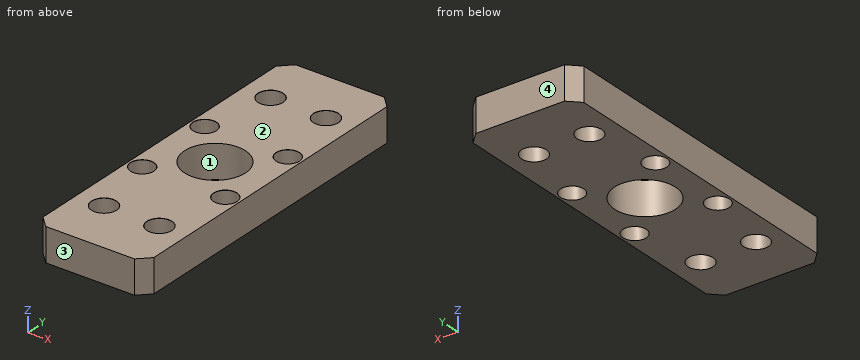
```python
from build123d import *

# Parameters (mm, degrees)
SKETCH_1_W                        = 20
SKETCH_1_H                        = 60
EXTRUDE_1_DEPTH                   = 6
HOLE_WIZARD_4_5_4_5_1_D           = 4.5
HOLE_WIZARD_4_5_4_5_1_CSINK_D     = 4.55
HOLE_WIZARD_4_5_4_5_1_CSINK_ANGLE = 90
SKETCH_4_R                        = 5.5
CUT_EXTRUDE_1_DEPTH               = 6
HOLE_WIZARD_4_2_4_2_1_D           = 4.2
HOLE_WIZARD_4_2_4_2_1_CSINK_D     = 4.25
HOLE_WIZARD_4_2_4_2_1_CSINK_ANGLE = 90
CHAMFER_1_SIZE                    = 2


with BuildPart() as part:
    # 草图1 → 凸台-拉伸1 (new body)
    with BuildSketch(Plane.XY):
        Rectangle(SKETCH_1_W, SKETCH_1_H)
    extrude(amount=EXTRUDE_1_DEPTH)

    # Ø4.5 (4.5) 直径孔1 (through all)
    with Locations(Plane(origin=(-5, 20, 6), x_dir=(1, 0, 0), z_dir=(0, 0, 1))):
        with Locations((0, 0), (10, 0)):
            hole_wizard_4_5_4_5_1 = CounterSinkHole(HOLE_WIZARD_4_5_4_5_1_D / 2, HOLE_WIZARD_4_5_4_5_1_CSINK_D / 2, counter_sink_angle=HOLE_WIZARD_4_5_4_5_1_CSINK_ANGLE)

    # 镜向1: Ø4.5 (4.5) 直径孔1 across plane
    add(hole_wizard_4_5_4_5_1.mirror(Plane.ZX), mode=Mode.SUBTRACT)

    # 草图4 → 切除-拉伸1 (cut)
    with BuildSketch(Plane.XY.offset(6)):
        Circle(SKETCH_4_R)
    extrude(amount=-CUT_EXTRUDE_1_DEPTH, mode=Mode.SUBTRACT)

    # Ø4.2 (4.2) 直径孔1 (through all)
    with Locations(Plane(origin=(-7.5, 7.5, 6), x_dir=(1, 0, 0), z_dir=(0, 0, 1))):
        with Locations((0, 0), (15, 0), (15, -15), (0, -15)):
            CounterSinkHole(HOLE_WIZARD_4_2_4_2_1_D / 2, HOLE_WIZARD_4_2_4_2_1_CSINK_D / 2, counter_sink_angle=HOLE_WIZARD_4_2_4_2_1_CSINK_ANGLE)

    # 倒角1
    chamfer_1_edges = [part.edges().sort_by_distance(p)[0] for p in [
        (10, -30, 3),
        (-10, -30, 3),
        (-10, 30, 3),
        (10, 30, 3),
    ]]
    chamfer(chamfer_1_edges, length=CHAMFER_1_SIZE)


solid = part.part
```
Geometry: final body of the model. Coordinates: model frame, mm. Face numbers are marked on the shaded views. Round coordinates to 2 decimals unless told otherwise and drop trailing zeros. Write each loop counter-clockwise with the first axis right and the second up, starting at its lowest first coordinate (ties: lowest second). Pieces come first, ordered by that corner, then holes.
Item 1: Section query A-A (y = -20). Return loops of the section in (x, z) (3 decimals), plus the area to 3 significant figures.
Item 2: Mould query, pull axis Y, two halves, no side actions, for the marked faces 1, 2, 3 and 4. Classes: +Y half, -Y half, draft (parallel to the pull), parting line (faces both ways), or undercut.
Item 3: Pin query (flat end, axial travel): P1, Ø5, axis at x = -7.5, y = -7.5, coming from the -Z side; P2, Ø4, axis at x = 7.5, y = -7.5, coming from the +Z side (1 decimal). Return the tip coordinate at first contact, or that it passes through.
Item 4: Section query D-D (y = 0). Return loops of the section in (x, z), plus the area to 3 significant figures.
Item 5: Section query B-B (x = 0). Return loops of the section in (y, z).
Item 6: Section query C-C (z = 5.3). Give the number of separate pieces and of enclosed holes in the cut face, plus the area to 3 significant figures.
Item 7: Material intervals for L1, parallel to X at y = -7.5, z = 1.3; L2, parallel to X at y = 20, z = 4; L3, parallel to Y at x = 7.5, z = 0.85, sorted ascending.
Completed:
1. outline: (-10, 0) - (-7.25, 0) - (-7.25, 5.975) - (-7.275, 6) - (-10, 6) - close; (-2.75, 0) - (2.75, 0) - (2.75, 5.975) - (2.725, 6) - (-2.725, 6) - (-2.75, 5.975) - close; (7.25, 0) - (10, 0) - (10, 6) - (7.275, 6) - (7.25, 5.975) - close
1. area: 66.0 mm2
2. face 1: undercut
2. face 2: draft
2. face 3: -Y half
2. face 4: +Y half
3. P1: stops at z = 0
3. P2: passes through
4. outline: (-10, 0) - (-5.5, 0) - (-5.5, 6) - (-10, 6) - close; (5.5, 0) - (10, 0) - (10, 6) - (5.5, 6) - close
4. area: 54.0 mm2
5. outline: (-30, 0) - (-5.5, 0) - (-5.5, 6) - (-30, 6) - close; (5.5, 0) - (30, 0) - (30, 6) - (5.5, 6) - close
6. separate pieces: 1
6. enclosed holes: 9
6. area: 978 mm2
7. L1: x = -10 to -9.6, -5.4 to 5.4, 9.6 to 10
7. L2: x = -10 to -7.25, -2.75 to 2.75, 7.25 to 10
7. L3: y = -30 to -9.6, -5.4 to 5.4, 9.6 to 30
